Model file for the job. Use its own axes, mm. A direction names the side the tool comes from. Give positions to 0.01 mm unless a question says otherwise; leave off trailing zeros. Write each loop counter-clockwise with the first axis right and the second up, starting at its lowest first coordinate (ties: lowest second). Pieces come first, ordered by that corner, then holes. Notation, with made-up numbers: (53, -20.5) - (61, -20.5) arc R13 ccw to (61, -2.5) - close; hole circle Ø5 at (74, 44). An arc over 180 degrees is marked (long way). One line per item, written item: value. Start each with the question number.
(1) Probe L1, parallel to Y at x = 0, z = 1.6; L2, parallel to Y at x = 0, z = 19.25; L3, parallel to Y at x = 0, z = 12. List the from-to ranges inside material, lowest first.
(2) Drop flat-ended pins along their axis: P1, Ø1.5, axis at x = -3, z = 11.5, coming from the +Y side; P2, Ø3, axis at x = -3, z = 21, coming from the +Y side; P3, Ø6, axis at y = 7, z = 9, coming from the +X side. Give the stop position or say it passes through.
(3) Mould opens along Y. For faces 3 (the face through (0, 9, 0)), 4 (the face through (0.1, 4.5, 13.8)), 5 (the face through (-0.215, 19.636, 1.479)) say: pulls with the +Y half, pulls with the -Y half, needs draft (parallel to the pull), parting line crosses it, or undercut.
(4) Cut at D-D, the plane z = 22.5. List the corners of the cut face in (x, y), and give its area (3 significant figures).
(5) Cut at A-A, the plane z = 2.5. List the corners of the cut face in (x, y).
(6) Cut at B-B, the plane x = 1. List the corners of the cut face in (y, z), and give its area (3 significant figures).
(7) Cut at C-C, the plane y = -1.5. List the corners of the cut face in (x, z), and give its area (3 significant figures).
(8) 3-axis set-ups, long thin cutter, end or side, ignore diameter. For faces 1 (the face through (0, 22, 1)), 2 (the face through (0, 2, 7)): which of +Z, -Z, +X, -X, +Y, -Y reach the whole face in a straight line?
from build123d import *

# Parameters (mm, degrees)
SKETCH_1_R          = 1.65
EXTRUDE_3_DEPTH     = 3
EXTRUDE_5_DEPTH     = 25
CUT_EXTRUDE_START   = 15
CUT_EXTRUDE_1_DEPTH = 10


with BuildPart() as part:
    # 草图1 → 凸台-拉伸3 (new body)
    with BuildSketch(Plane.XY):
        with BuildLine():
            ThreePointArc((-4.5, 0), (0, -4.5), (4.5, 0))
            Line((4.5, 0), (4, 18))
            ThreePointArc((4, 18), (0, 22), (-4, 18))
            Line((-4, 18), (-4.5, 0))
        make_face()
        with Locations((0, 18)):
            Circle(SKETCH_1_R, mode=Mode.SUBTRACT)
        with BuildLine():
            Line((-1.887458609, 2), (1.887458609, 2))
            ThreePointArc((1.887458609, 2), (0, -2.75), (-1.887458609, 2))
        make_face(mode=Mode.SUBTRACT)
    extrude(amount=EXTRUDE_3_DEPTH)

    # 草图1<12> → 凸台-拉伸5 (add)
    with BuildSketch(Plane.XY):
        with BuildLine():
            Line((-4.49306091, 0.249807247), (-4.5, 0))
            ThreePointArc((-4.5, 0), (0, -4.5), (4.5, 0))
            Line((4.5, 0), (4.49306091, 0.249807247))
            ThreePointArc((4.49306091, 0.249807247), (0, 4.5), (-4.49306091, 0.249807247))
        make_face()
        with BuildLine():
            Line((-1.887458609, 2), (1.887458609, 2))
            ThreePointArc((1.887458609, 2), (0, -2.75), (-1.887458609, 2))
        make_face(mode=Mode.SUBTRACT)
    extrude(amount=EXTRUDE_5_DEPTH)

    # 草图1<16> → 切除-拉伸1 (cut)
    with BuildSketch(Plane.XY.offset(CUT_EXTRUDE_START)):
        with BuildLine():
            ThreePointArc((0, 2.75), (-1.015504801, 2.555631038), (-1.887458609, 2))
            Line((-1.887458609, 2), (0, 2))
            Line((0, 2), (0, 2.75))
        make_face()
        with BuildLine():
            Line((0, 2), (-1.887458609, 2))
            ThreePointArc((-1.887458609, 2), (-2.555631038, -1.015504801), (0, -2.75))
            Line((0, -2.75), (0, 2))
        make_face()
        with BuildLine():
            Line((0, 2.75), (0, 2))
            Line((0, 2), (1.887458609, 2))
            ThreePointArc((1.887458609, 2), (1.015504801, 2.555631038), (0, 2.75))
        make_face()
        with BuildLine():
            Line((1.887458609, 2), (0, 2))
            Line((0, 2), (0, -2.75))
            ThreePointArc((0, -2.75), (1.944543648, -1.944543648), (2.75, 0))
            ThreePointArc((2.75, 0), (2.525174368, 1.089033706), (1.887458609, 2))
        make_face()
    extrude(amount=CUT_EXTRUDE_1_DEPTH, mode=Mode.SUBTRACT)


solid = part.part
Answers follow:
1. L1: y = -4.5 to -2.75, 2 to 16.35, 19.65 to 22
1. L2: y = -4.5 to -2.75, 2.75 to 4.5
1. L3: y = -4.5 to -2.75, 2 to 4.5
2. P1: stops at y = 3.9
2. P2: stops at y = 4.24
2. P3: stops at x = 2.06
3. face 3: needs draft
3. face 4: pulls with the +Y half
3. face 5: undercut
4. outline: (-4.5, 0) arc R4.5 ccw to (4.5, 0) - (4.49, 0.25) arc R4.5 ccw to (-4.49, 0.25) - close; hole circle Ø5.5 at (0, 0)
4. area: 39.9 mm²
5. outline: (-4.5, 0) arc R4.5 ccw to (4.5, 0) - (4, 18) arc R4 ccw to (-4, 18) - close; hole (-1.89, 2) arc R2.75 ccw (long way) to (1.89, 2) - close; hole circle Ø3.3 at (0, 18)
6. outline: (-4.39, 0) - (-2.56, 0) - (-2.56, 25) - (-4.39, 25) - close; (2, 0) - (16.69, 0) - (16.69, 3) - (4.39, 3) - (4.39, 25) - (2.56, 25) - (2.56, 15) - (2, 15) - close; (19.31, 0) - (21.87, 0) - (21.87, 3) - (19.31, 3) - close
6. area: 144 mm²
7. outline: (-4.24, 0) - (-2.3, 0) - (-2.3, 25) - (-4.24, 25) - close; (2.3, 0) - (4.24, 0) - (4.24, 25) - (2.3, 25) - close
7. area: 96.9 mm²
8. face 1: +Z, -Z, +Y
8. face 2: +Z, -Z
